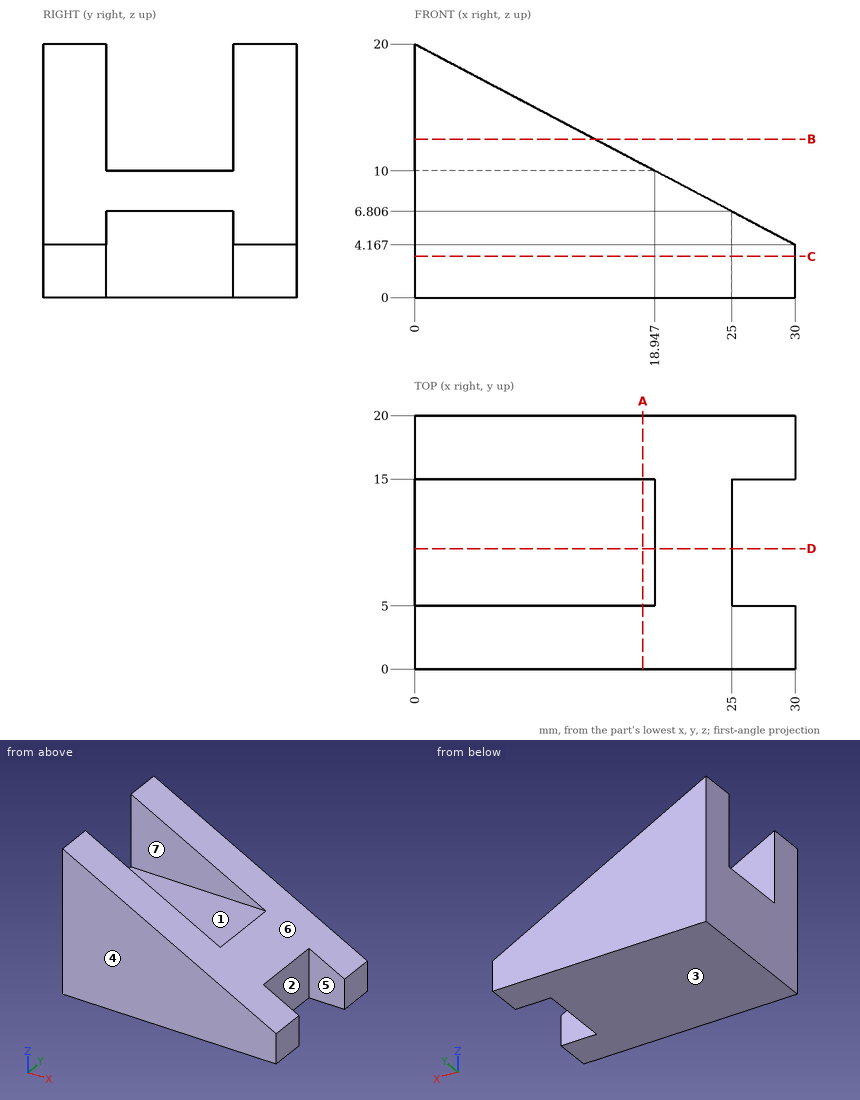
Verification items for this drawing (mm, ordinates from the low corner). A direction names the side the tool comes from. Give positions to 0.01 mm unless a question says otherwise; leave off trailing zeros. Loops run counter-clockwise (first coordinate to the right, second up) from the corner with the lowest first, then second, coordinate; pieces in that order, holes last. Notation, with made-up numbers: M 86,7.5 L 144,7.5 A18 cw 144,22.5 Z; hole C -31.5,-18.75 d6. An arc over 180 degrees is marked long. Write item = value, one per line. Start each with the question number.
1. Section check B-B, the plane z = 12.5. Enter the section's corners in (x, y).
2. Section check C-C, the plane z = 3.25. Enter the section's corners in (x, y).
3. Section check A-A, the plane x = 18. Enter the section's corners in (y, z).
4. Tool access check on the marked faces 1, 2 and 3. Record the directions out of +Z, -Z, +X, -X, +Y, -Y that give a thin tool (end or side, any length) a straight path to the whole face; none if there is none.
5. Go/stop test with flat-tipped pins: P1, Ø12, axis at y = 14, z = 11, coming from the +X side (1 decimal); P2, Ø3.5, axis at y = 10.5, z = 4.5, coming from the +X side. Record where each tip stops, or that it passes through.
6. Section check D-D, the plane y = 9.5. Enter the section's corners in (x, z) (1 decimal), plus the area to 3 significant figures.
7. Draft check along Y on the marked faces 4, 5, 6 and 7. Enter one of: +Y half, -Y half, draft (parallel to the pull), parting line (faces both ways), or undercut.
8. Thickness scan on probe 1 along X at (y, z) = (5.75, 3.5); probe 2 along Z at (x, y) = (11.75, 9.75); probe 3 along X at (y, z) = (14.5, 9) (1 decimal). Record the ranges inside material, lowest first.
Values follow:
q1.outline = M 0,0 L 14.21,0 L 14.21,5 L 0,5 Z; M 0,15 L 14.21,15 L 14.21,20 L 0,20 Z
q2.outline = M 0,0 L 30,0 L 30,5 L 25,5 L 25,15 L 30,15 L 30,20 L 0,20 Z
q3.outline = M 0,0 L 20,0 L 20,10.5 L 15,10.5 L 15,10 L 5,10 L 5,10.5 L 0,10.5 Z
q4.face_1 = +Z, +X, -X
q4.face_2 = +Z, -Z, +X
q4.face_3 = -Z, +X, -X, +Y, -Y
q5.P1 = 28.3
q5.P2 = 25
q6.outline = M 0,0 L 25,0 L 25,6.8 L 18.9,10 L 0,10 Z
q6.area = 240 mm^2
q7.face_4 = -Y half
q7.face_5 = undercut
q7.face_6 = draft
q7.face_7 = undercut
q8.probe_1 = 0 to 25
q8.probe_2 = 0 to 10
q8.probe_3 = 0 to 20.8
